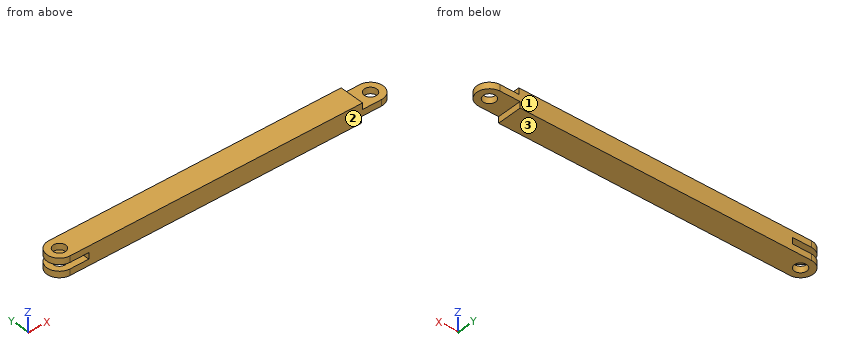
from build123d import *

# Parameters (mm, degrees)
SKETCH1_R           = 10
BOSS_EXTRUDE1_DEPTH = 30
SKETCH4_W           = 69.930145124
SKETCH4_H           = 10
CUT_EXTRUDE1_DEPTH  = 523.398315464


with BuildPart() as part:
    # Sketch1 → Boss-Extrude1 (new body)
    with BuildSketch(Plane.XY):
        with BuildLine():
            Line((0, 20), (500, 20))
            ThreePointArc((500, 20), (520, 0), (500, -20))
            Line((500, -20), (0, -20))
            ThreePointArc((0, -20), (-20, 0), (0, 20))
        make_face()
        Circle(SKETCH1_R, mode=Mode.SUBTRACT)
        with Locations((500, 0)):
            Circle(SKETCH1_R, mode=Mode.SUBTRACT)
    extrude(amount=BOSS_EXTRUDE1_DEPTH)

    # Sketch4 → Cut-Extrude1 (cut, through all)
    with BuildSketch(Plane.XZ.offset(20)):
        with Locations((-4.965072562, 15)):
            Rectangle(SKETCH4_W, SKETCH4_H)
        Polygon((470, 47.162996114), (470, 20), (535.290811534, 20), (535.290811534, 10), (467.990842664, 10), (467.990842664, -15.795499521), (553.153388579, -15.795499521), (553.153388579, 47.162996114), align=None)
    extrude(amount=-CUT_EXTRUDE1_DEPTH, mode=Mode.SUBTRACT)


solid = part.part
Geometry: final body of the model. Coordinates: model frame, mm. Face numbers are marked on the shaded views. Coordinates: 2 decimals unless noted, no trailing zeros. One line per item, written item: value. Start each with the question number.
1) Draft query along Y for the marked faces 1, 2 and 3. Return one class per face: released by +Y, released by -Y, zero draft, split by the parting line, or undercut.
2) Material intervals for L1, parallel to Y at x = 0, z = 24.25; L2, parallel to X at y = 0, z = 26.5; L3, parallel to X at y = 0, z = 6.5, sorted ascending. Write a range as from..to.
3) Pin query (flat end, axial travel): P1, Ø2, axis at y = 1.5, z = 8, coming from the -X side; P2, Ø12, axis at x = 497.5, y = 10, coming from the +Z side; P3, Ø3, axis at y = 11.5, z = 19, coming from the -X side. Return the tip coordinate at first contact, or that it passes through.
Evaluation:
1. face 1: released by +Y
1. face 2: released by -Y
1. face 3: zero draft
2. L1: -20..-10, 10..20
2. L2: -20..-10, 10..470
2. L3: -20..-10, 10..467.99
3. P1: x = -19.99
3. P2: z = 20
3. P3: x = -17.09
